Geometry check sheet. Reference: the model listing, model coordinates, mm. A direction names the side the tool comes from. Round coordinates to 2 decimals unless told otherwise and drop trailing zeros. Order: outer loops, then holes, each group sorted by start corner. A loop starts at its lowest first (then second) coordinate and runs counter-clockwise, first axis right, second up. Notation, with made-up numbers: M 6,57 L 55,57 A21 ccw 55,94 Z; hole C -19.5,76 d4. An arc over 180 degrees is marked long. Answer as a JSON object with one key per item and string values. Group by question number.
Autodesk Inventor part; units mm, degrees
ref_plane "Plano de trabajo1" through (0, 10, 0) normal (0, 1, 0) x (1, 0, 0)
ref_plane "Plano de trabajo4" through (0, -3, 0) normal (0, -1, 0) x (1, 0, 0)
ref_plane "Plano de trabajo5" through (20, -33, 15) normal (0, 0, -1) x (-1, 0, 0)
ref_plane "Plano de trabajo1" through (0, 10, 0) normal (0, 1, 0) x (1, 0, 0)
sketch "Boceto3" plane through (0, 10, 0) normal (0, 1, 0) x (1, 0, 0)
  line L0 (20, -20) -> (0, -20)
  line L1 (0, 0) -> (20, 0)
  line L2 (0, -20) -> (20, -20)
  line L3 (20, -20) -> (20, 0)
  line L4 (20, 0) -> (0, 0)
  line L5 (0, 0) -> (0, -20)
extrude "Extrusión3" add sketch "Boceto3" along normal blind 5
ref_plane "Plano de trabajo4" through (0, -3, 0) normal (0, -1, 0) x (1, 0, 0)
sketch "Boceto8" plane through (0, -3, 0) normal (0, -1, 0) x (1, 0, 0)
  line L0 (0, 0) -> (0, 20)
  line L1 (0, 20) -> (20, 20)
  line L2 (0, 15) -> (20, 15)
  line L3 (20, 15) -> (20, 20)
  line L4 (20, 20) -> (0, 20)
  line L5 (0, 20) -> (0, 15)
  dimension "d25" = 5
extrude "Extrusión8" add sketch "Boceto8" along normal blind 30
ref_plane "Plano de trabajo5" through (20, -33, 15) normal (0, 0, -1) x (-1, 0, 0)
sketch "Boceto10" plane through (20, -33, 15) normal (0, 0, -1) x (-1, 0, 0)
  circle A0 centre (10, 17.2) radius 3.15
  line L0 (0, 33) -> (20, 33)
  line L1 (0, 32) -> (0, 0)
  point P0 (15.75, 33)
  point P1 (10, 33)
  dimension "d35" = 6.3
  dimension "d36" = 15.8
  dimension "d37" = 10
extrude "Extrusión9" add sketch "Boceto10" along normal blind 15
ref_plane "Plano de trabajo2" through (20, 10, 20) normal (1, 0, 0) x (0, 0, -1)
sketch "Boceto13" plane through (0, -3, 0) normal (0, 1, 0) x (1, 0, 0)
  line L0 (0, -20) -> (0, -15)
  line L1 (20, -15) -> (20, -20)
  line L2 (0, -15) -> (20, -15)
  line L3 (20, -15) -> (20, -20)
  line L4 (20, -20) -> (0, -20)
  line L5 (0, -20) -> (0, -15)
  point P0 (0, 0)
extrude "Extrusión12" add sketch "Boceto13" along normal blind 13
sketch "Boceto15" plane through (0, 15, 0) normal (0, 1, 0) x (1, 0, 0)
  circle A0 centre (10, -10) radius 2.5
  line L0 (0, 0) -> (0, -20)
  line L1 (0, -20) -> (20, -20)
  point P0 (320, -20)
  dimension "d58" = 5
  dimension "d59" = 10
  dimension "d60" = 10
extrude "Extrusión14" cut sketch "Boceto15" against normal blind 5
sketch "Boceto16" plane through (0, 10, 0) normal (-1, 0, 0) x (0, 0, 1)
  line L0 (20, 5) -> (0, 5)
  line L1 (20, 5) -> (20, -43)
  line L2 (0, 5) -> (20, 5)
  line L3 (20, 5) -> (20, 0)
  line L4 (20, 0) -> (0, 0)
  line L5 (0, 0) -> (0, 5)
  point P0 (0, -10)
  dimension "d63" = 5
extrude "Extrusión15" add sketch "Boceto16" along normal blind 300
sketch "Boceto18" plane through (0, 15, 0) normal (0, 1, 0) x (1, 0, 0)
  circle A0 centre (-290, -10) radius 2.5
  line L0 (20, -20) -> (-300, -20)
  line L1 (-300, -20) -> (-300, 0)
  point P0 (0, 0)
  dimension "d66" = 5
  dimension "d67" = 10
  dimension "d68" = 10
extrude "Extrusión16" cut sketch "Boceto18" against normal blind 300
sketch "Boceto19" plane through (0, 15, 0) normal (0, 1, 0) x (1, 0, 0)
  circle A0 centre (-275, -10) radius 2.5
  circle A1 centre (-290, -10) radius 2.5
  point P0 (0, 0)
  dimension "d71" = 5
  dimension "d72" = 0
  dimension "d73" = 15
extrude "Extrusión17" cut sketch "Boceto19" against normal blind 10 contours A0
thread "Rosca4"
thread "Rosca5"
thread "Rosca6"
properties part number "Ejes Base - C15_3DPrint"
1) Sectioned sample at A-A (z = 3.25). Record the boundary of the cut face in (x, y), then the cut area to 3 significant figures.
2) Thickness scan on line 1 along X through (y, z) = (12.9, 10); line 2 along Y through (x, z) = (-261, 6.5); line 3 along Z through (x, y) = (-275, 11.75). Record the ranges inside material, lowest first. Write a range as [from, to].
3) Sectioned sample at B-B (x = -72). Record the boundary of the cut face in (y, z), then the cut area to 3 significant figures.
4) Set-up check for faces 1 (the cylindrical face through (12.32, -17.93, 7.6)), 2 (the flat face through (10, -16, 0)), 3 (the flat face through (0, -12, 17)): record each of +Z, -Z, +X, -X, +Y, -Y from which the full face is reachable in a straight line by a thin tool's end or side.
5) Sectioned sample at C-C (y = 2). Record the boundary of the cut face in (x, z), then the cut area to 3 significant figures.
6) Release check for a two-part mould opening along Z. For faces 4 (the flat face through (10, -12, 15)), 5 (the cylindrical face through (9.46, 12.54, 12.44)), 6 (the flat face through (20, -3.8, 15.2)) record: +Z half, -Z half, draft (parallel to the pull), parting line (faces both ways), or undercut.
7) Go/stop test with flat-tipped pins: P1, Ø1.5, axis at y = -9, z = 18.5, coming from the -X side; P2, Ø6, axis at x = -290, z = 10, coming from the +Y side; P3, Ø5, axis at x = -185, z = 17.5, coming from the -Y side; P4, Ø4, axis at y = -19.5, z = 12.5, coming from the +X side. Record where each tip stops, or that it passes through.
Final values:
{
 "1": {"outline": "M -300,10 L 20,10 L 20,15 L -300,15 Z; C 10,-15.8 d6.3", "area": "1,630 mm^2"},
 "2": {"line 1": "x = [-300, -292.5], [-287.5, -277.5], [-272.5, 7.5], [12.5, 20]", "line 2": "y = [10, 15]", "line 3": "z = [0, 7.5], [12.5, 20]"},
 "3": {"outline": "M 10,0 L 15,0 L 15,20 L 10,20 Z", "area": "100 mm^2"},
 "4": {"face 1": "-Z", "face 2": "-Z, +X, -X, +Y, -Y", "face 3": "+Z, -Z, -X, -Y"},
 "5": {"outline": "M 0,15 L 20,15 L 20,20 L 0,20 Z", "area": "100 mm^2"},
 "6": {"face 4": "-Z half", "face 5": "undercut", "face 6": "draft"},
 "7": {"P1": "stops at x = 0", "P2": "stops at y = 15", "P3": "stops at y = 10", "P4": "stops at x = 12.65"}
}
